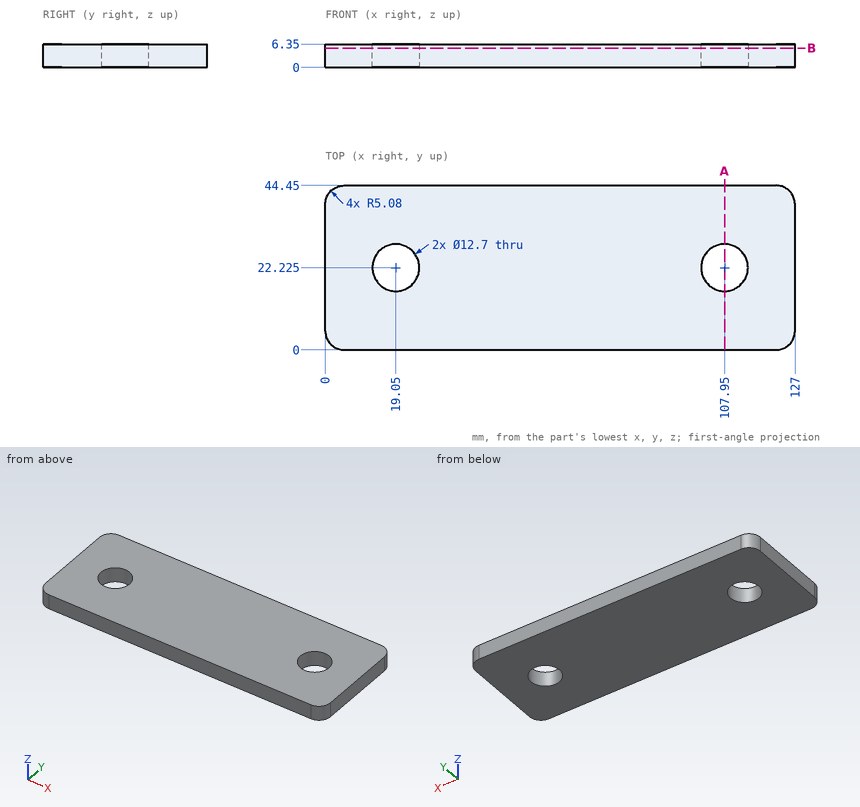
Study the drawing (mm; zero at the part's minimum x, y, z) and answer. Round coordinates to 2 decimals unless told otherwise and drop trailing zeros. Loops run counter-clockwise (first coordinate to the right, second up) from the corner with the lowest first, then second, coordinate; pieces in that order, holes last. Notation, with made-up numbers: (50.5, 84.5) - (106.5, 84.5) arc R32 ccw to (106.5, 115.5) - close; hole circle Ø10 at (0, 4.25). An arc over 180 degrees is marked (long way). Use one line per item in the form item = value. Start each with the question number.
1. The part is cut by section A-A on x = 107.95. Determine the outline of the cut face in (y, z) (3 decimals), then the cut area to 3 significant figures.
2. The part is cut by section B-B on z = 5.25. Determine the outline of the cut face in (x, y) (3 decimals).
3. Consider line 1 (Y direction, x = 107.95, z = 2.75) (3 decimals); line 2 (X direction, y = 18, z = 3); line 3 (X direction, y = 19, z = 4). Determine where each line is inside the solid, lowest interval first. Write a range as [from, to].
Geometry check:
q1.outline = (0, 0) - (15.875, 0) - (15.875, 6.35) - (0, 6.35) - close; (28.575, 0) - (44.45, 0) - (44.45, 6.35) - (28.575, 6.35) - close
q1.area = 202 mm^2
q2.outline = (0, 5.08) arc R5.08 ccw to (5.08, 0) - (121.92, 0) arc R5.08 ccw to (127, 5.08) - (127, 39.37) arc R5.08 ccw to (121.92, 44.45) - (5.08, 44.45) arc R5.08 ccw to (0, 39.37) - close; hole circle Ø12.7 at (19.05, 22.225); hole circle Ø12.7 at (107.95, 22.225)
q3.line_1 = [0, 15.875], [28.575, 44.45]
q3.line_2 = [0, 14.31], [23.79, 103.21], [112.69, 127]
q3.line_3 = [0, 13.58], [24.52, 102.48], [113.42, 127]
